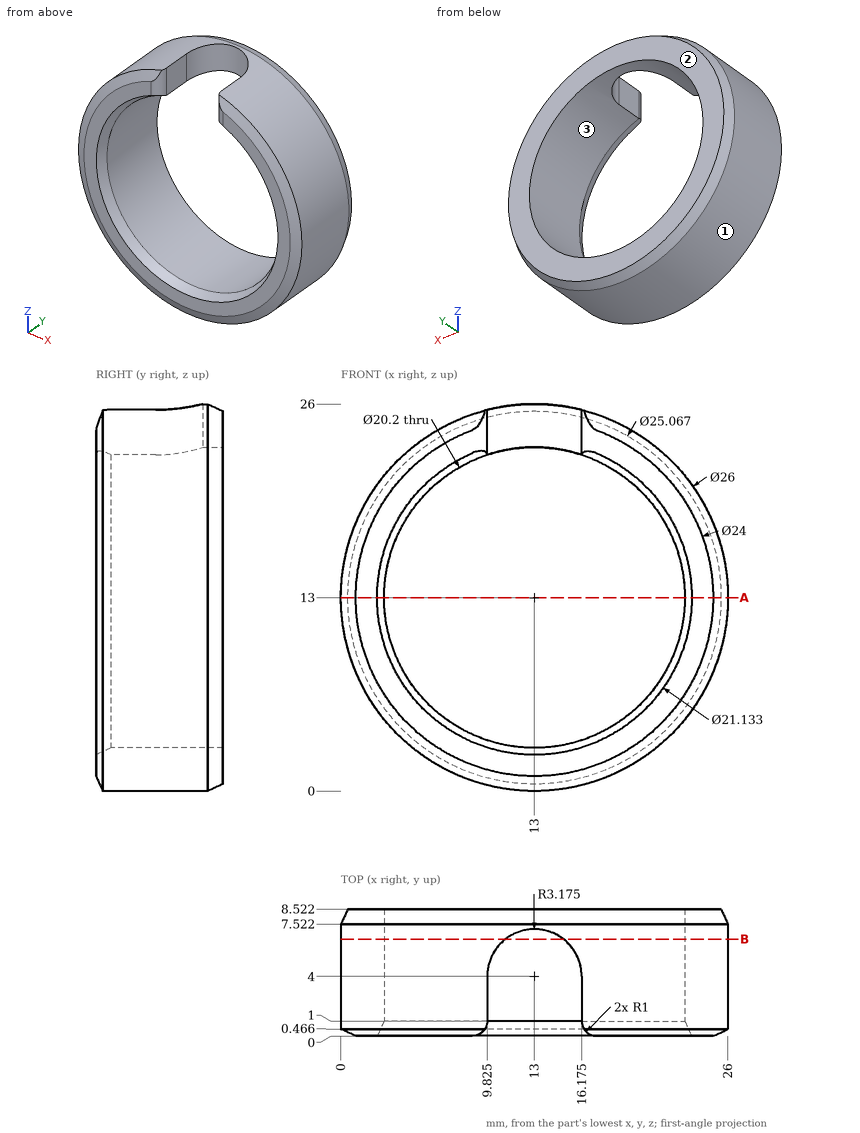
Here's the drawing with two shaded views (mm, measured from the low corner). I have some questions. Give positions to 0.01 mm unless a question says otherwise; leave off trailing zeros. Write each loop counter-clockwise with the first axis right and the second up, starting at its lowest first coordinate (ties: lowest second). Pieces come first, ordered by that corner, then holes. Notation, with made-up numbers: (83, -29.75) - (132, -29.75) arc R23 cw to (132, -16.75) - close; hole circle Ø7 at (53, 33.25). An arc over 180 degrees is marked (long way). Write item = value, one per line. Start each with the question number.
1. Imagine slicing it at A-A (z = 13). Please give me the cut outline in (x, y).
2. For pin 1 (1.5 mm diameter, centred on y = 2.5, z = 23.5, fed in from -X); pin 2 (2.5 mm diameter, centred on y = 2.5, z = 24.5, fed in from +X) (1 decimal); pin 3 (3 mm diameter, centred on x = 21, y = 2, fed in from -Z), each with a flat end and sliding along its axis, tell me the tip position at first contact or that it passes through.
3. Thinking about a two-plate mould opening in X: for the marked faces 1, 2 and 3, which applies, released by +X, released by -X, zero draft, split by the parting line, or undercut?
4. Please list where these lines run through material, in increasing order: line 1 (X direction, y = 4.25, z = 13); line 2 (Z direction, x = 13, y = 2.5); line 3 (X direction, y = 2.5, z = 3.75) (1 decimal).
5. Imagine slicing it at B-B (y = 6.5). Please give me the cut outline in (x, z).
Worked answers:
q1.outline = (0, 0.47) - (1, 0) - (2.43, 0) - (2.9, 1) - (2.9, 8.52) - (0.47, 8.52) - (0, 7.52) - close; (23.1, 1) - (23.57, 0) - (25, 0) - (26, 0.47) - (26, 7.52) - (25.53, 8.52) - (23.1, 8.52) - close
q2.pin_1 = 4.4
q2.pin_2 = 21
q2.pin_3 = 1.74
q3.face_1 = split by the parting line
q3.face_2 = zero draft
q3.face_3 = undercut
q4.line_1 = 0 to 2.9, 23.1 to 26
q4.line_2 = 0 to 2.9
q4.line_3 = 3.9 to 8.9, 17.1 to 22.1
q5.outline = (11.04, 22.91) - (11.04, 25.85) arc R13 ccw (long way) to (14.96, 25.85) - (14.96, 22.91) arc R10.1 cw (long way) to start
